Verification items for this drawing (mm, ordinates from the low corner). Round coordinates to 2 decimals unless told otherwise and drop trailing zeros. Order: outer loops, then holes, each group sorted by start corner. A loop starts at its lowest first (then second) coordinate and runs counter-clockwise, first axis right, second up. Notation, with made-up numbers: (2.5, 85.5) -> (13.5, 85.5) arc R23 cw to (13.5, 119.5) -> close; hole circle Ø1 at (-26.5, 33.25). An arc over 180 degrees is marked (long way). Answer in a Markdown table with one row per item. Add a question column.
1. Sectioned sample at A-A, the plane x = 8.25. Record the boundary of the cut face in (y, z) (3 decimals).
2. Draft check along X on the marked faces 1, 2, 3 and 4. Enter one of: +X half, -X half, draft (parallel to the pull), parting line (faces both ways), or undercut.
3. Sectioned sample at B-B, the plane z = 4.5. Record the boundary of the cut face in (x, y), then the cut area to 4 significant figures.
4. Material ranges on L1, parallel to Y at x = 8.75, z = 7.25, recorded low to high. Write a range as from..to.
5. Depth check by flat-ended pin: P1, Ø0.6, axis at x = 0.5, z = 3, coming from the -Y side; P2, Ø0.6, axis at x = 5.5, y = 1, coming from the -Z side (3 decimals); P3, Ø0.6, axis at x = 8.5, y = 2.5, coming from the +Z side (3 decimals). Enter the tip coordinate at first touch or a pass-through.
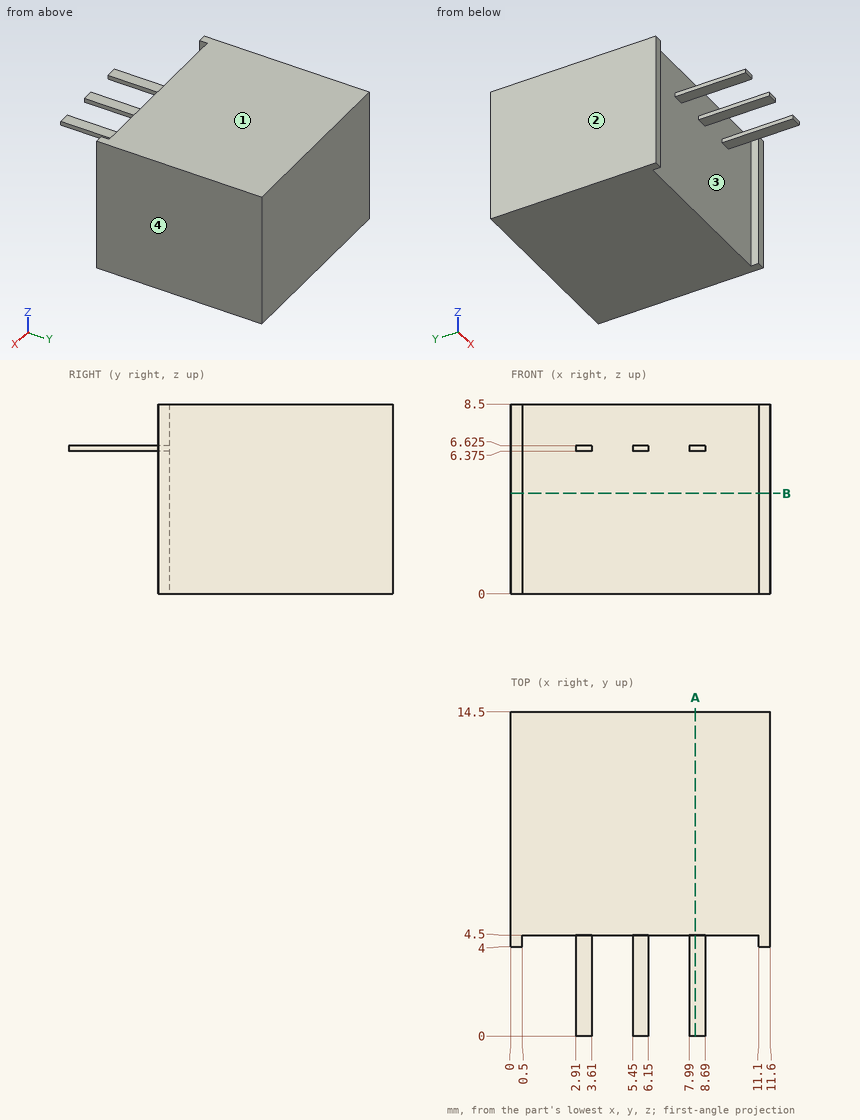
Answer key:
| question | item | result |
|---|---|---|
| 1 | outline | (0, 6.375) -> (4.5, 6.375) -> (4.5, 0) -> (14.5, 0) -> (14.5, 8.5) -> (4.5, 8.5) -> (4.5, 6.625) -> (0, 6.625) -> close |
| 2 | face 1 | draft |
| 2 | face 2 | -X half |
| 2 | face 3 | undercut |
| 2 | face 4 | +X half |
| 3 | outline | (0, 4) -> (0.5, 4) -> (0.5, 4.5) -> (11.1, 4.5) -> (11.1, 4) -> (11.6, 4) -> (11.6, 14.5) -> (0, 14.5) -> close |
| 3 | area | 116.5 mm² |
| 4 | L1 | y = 4.5..14.5 |
| 5 | P1 | stops at y = 4 |
| 5 | P2 | stops at z = 6.375 |
| 5 | P3 | stops at z = 6.625 |
